Verification items for the finished model (mm, model axes). A direction names the side the tool comes from. Round coordinates to 2 decimals unless told otherwise and drop trailing zeros. Write each loop counter-clockwise with the first axis right and the second up, starting at its lowest first coordinate (ties: lowest second). Pieces come first, ordered by that corner, then holes. Notation, with made-up numbers: M 26,55 L 42,55 A21 cw 42,84 Z; hole C 24.5,-32 d8. An arc over 180 degrees is marked long. Write each question's results on one line, items separated by ' | '.
from build123d import *

# Parameters (mm, degrees)
PAD_DEPTH       = 250
POCKET_DEPTH    = 2
POCKET001_DEPTH = 3


with BuildPart() as part:
    # Sketch → Pad (new body)
    with BuildSketch(Plane.XZ):
        Polygon((0, 0), (-15, 0), (-15, 1.5), (-14, 1.5), (-14, 5.5), (-17.5, 6.5), (-17.5, 7.5), (-12.5, 7.5), (-12.5, 1.5), (0, 1.5), (12.5, 1.5), (12.5, 7.5), (17.5, 7.5), (17.51485, 6.5), (14, 5.5), (14, 1.5), (15, 1.5), (15, 0), align=None)
    extrude(amount=PAD_DEPTH)

    # Sketch001 (on Face10 of Pad) → Pocket (cut)
    with BuildSketch(Plane(origin=(0, 0, 1.5), x_dir=(-1, 0, 0), z_dir=(0, 0, 1))):
        with BuildLine():
            ThreePointArc((2.5, 2.5), (0, 5), (-2.5, 2.5))
            Line((-2.5, 2.5), (-2.5, -2.5))
            ThreePointArc((-2.5, -2.5), (0, -5), (2.5, -2.5))
            Line((2.5, 2.5), (2.5, -2.5))
        make_face()
        with BuildLine():
            ThreePointArc((2.5, 15), (0, 17.5), (-2.5, 15))
            Line((-2.5, 15), (-2.5, 10))
            ThreePointArc((-2.5, 10), (0, 7.5), (2.5, 10))
            Line((2.5, 15), (2.5, 10))
        make_face()
        with BuildLine():
            ThreePointArc((2.5, 27.5), (0, 30), (-2.5, 27.5))
            Line((-2.5, 27.5), (-2.5, 22.5))
            ThreePointArc((-2.5, 22.5), (0, 20), (2.5, 22.5))
            Line((2.5, 27.5), (2.5, 22.5))
        make_face()
        with BuildLine():
            ThreePointArc((2.5, 40), (0, 42.5), (-2.5, 40))
            Line((-2.5, 40), (-2.5, 35))
            ThreePointArc((-2.5, 35), (0, 32.5), (2.5, 35))
            Line((2.5, 40), (2.5, 35))
        make_face()
        with BuildLine():
            ThreePointArc((2.5, 52.5), (0, 55), (-2.5, 52.5))
            Line((-2.5, 52.5), (-2.5, 47.5))
            ThreePointArc((-2.5, 47.5), (0, 45), (2.5, 47.5))
            Line((2.5, 52.5), (2.5, 47.5))
        make_face()
        with BuildLine():
            ThreePointArc((2.5, 65), (0, 67.5), (-2.5, 65))
            Line((-2.5, 65), (-2.5, 60))
            ThreePointArc((-2.5, 60), (0, 57.5), (2.5, 60))
            Line((2.5, 65), (2.5, 60))
        make_face()
        with BuildLine():
            ThreePointArc((2.5, 77.5), (0, 80), (-2.5, 77.5))
            Line((-2.5, 77.5), (-2.5, 72.5))
            ThreePointArc((-2.5, 72.5), (0, 70), (2.5, 72.5))
            Line((2.5, 77.5), (2.5, 72.5))
        make_face()
        with BuildLine():
            ThreePointArc((2.5, 90), (0, 92.5), (-2.5, 90))
            Line((-2.5, 90), (-2.5, 85))
            ThreePointArc((-2.5, 85), (0, 82.5), (2.5, 85))
            Line((2.5, 90), (2.5, 85))
        make_face()
        with BuildLine():
            ThreePointArc((2.5, 102.5), (0, 105), (-2.5, 102.5))
            Line((-2.5, 102.5), (-2.5, 97.5))
            ThreePointArc((-2.5, 97.5), (0, 95), (2.5, 97.5))
            Line((2.5, 102.5), (2.5, 97.5))
        make_face()
        with BuildLine():
            ThreePointArc((2.5, 115), (0, 117.5), (-2.5, 115))
            Line((-2.5, 115), (-2.5, 110))
            ThreePointArc((-2.5, 110), (0, 107.5), (2.5, 110))
            Line((2.5, 115), (2.5, 110))
        make_face()
        with BuildLine():
            ThreePointArc((2.5, 127.5), (0, 130), (-2.5, 127.5))
            Line((-2.5, 127.5), (-2.5, 122.5))
            ThreePointArc((-2.5, 122.5), (0, 120), (2.5, 122.5))
            Line((2.5, 127.5), (2.5, 122.5))
        make_face()
        with BuildLine():
            ThreePointArc((2.5, 140), (0, 142.5), (-2.5, 140))
            Line((-2.5, 140), (-2.5, 135))
            ThreePointArc((-2.5, 135), (0, 132.5), (2.5, 135))
            Line((2.5, 140), (2.5, 135))
        make_face()
        with BuildLine():
            ThreePointArc((2.5, 152.5), (0, 155), (-2.5, 152.5))
            Line((-2.5, 152.5), (-2.5, 147.5))
            ThreePointArc((-2.5, 147.5), (0, 145), (2.5, 147.5))
            Line((2.5, 152.5), (2.5, 147.5))
        make_face()
        with BuildLine():
            ThreePointArc((2.5, 165), (0, 167.5), (-2.5, 165))
            Line((-2.5, 165), (-2.5, 160))
            ThreePointArc((-2.5, 160), (0, 157.5), (2.5, 160))
            Line((2.5, 165), (2.5, 160))
        make_face()
        with BuildLine():
            ThreePointArc((2.5, 177.5), (0, 180), (-2.5, 177.5))
            Line((-2.5, 177.5), (-2.5, 172.5))
            ThreePointArc((-2.5, 172.5), (0, 170), (2.5, 172.5))
            Line((2.5, 177.5), (2.5, 172.5))
        make_face()
        with BuildLine():
            ThreePointArc((2.5, 190), (0, 192.5), (-2.5, 190))
            Line((-2.5, 190), (-2.5, 185))
            ThreePointArc((-2.5, 185), (0, 182.5), (2.5, 185))
            Line((2.5, 190), (2.5, 185))
        make_face()
        with BuildLine():
            ThreePointArc((2.5, 202.5), (0, 205), (-2.5, 202.5))
            Line((-2.5, 202.5), (-2.5, 197.5))
            ThreePointArc((-2.5, 197.5), (0, 195), (2.5, 197.5))
            Line((2.5, 202.5), (2.5, 197.5))
        make_face()
        with BuildLine():
            ThreePointArc((2.5, 215), (0, 217.5), (-2.5, 215))
            Line((-2.5, 215), (-2.5, 210))
            ThreePointArc((-2.5, 210), (0, 207.5), (2.5, 210))
            Line((2.5, 215), (2.5, 210))
        make_face()
        with BuildLine():
            ThreePointArc((2.5, 227.5), (0, 230), (-2.5, 227.5))
            Line((-2.5, 227.5), (-2.5, 222.5))
            ThreePointArc((-2.5, 222.5), (0, 220), (2.5, 222.5))
            Line((2.5, 227.5), (2.5, 222.5))
        make_face()
        with BuildLine():
            ThreePointArc((2.5, 240), (0, 242.5), (-2.5, 240))
            Line((-2.5, 240), (-2.5, 235))
            ThreePointArc((-2.5, 235), (0, 232.5), (2.5, 235))
            Line((2.5, 240), (2.5, 235))
        make_face()
        with BuildLine():
            ThreePointArc((2.5, 252.5), (0, 255), (-2.5, 252.5))
            Line((-2.5, 252.5), (-2.5, 247.5))
            ThreePointArc((-2.5, 247.5), (0, 245), (2.5, 247.5))
            Line((2.5, 252.5), (2.5, 247.5))
        make_face()
        with BuildLine():
            ThreePointArc((2.5, 265), (0, 267.5), (-2.5, 265))
            Line((-2.5, 265), (-2.5, 260))
            ThreePointArc((-2.5, 260), (0, 257.5), (2.5, 260))
            Line((2.5, 265), (2.5, 260))
        make_face()
        with BuildLine():
            ThreePointArc((2.5, 277.5), (0, 280), (-2.5, 277.5))
            Line((-2.5, 277.5), (-2.5, 272.5))
            ThreePointArc((-2.5, 272.5), (0, 270), (2.5, 272.5))
            Line((2.5, 277.5), (2.5, 272.5))
        make_face()
        with BuildLine():
            ThreePointArc((-2.5, 285), (0, 282.5), (2.5, 285))
            Line((2.5, 285), (2.5, 290))
            ThreePointArc((2.5, 290), (0, 292.5), (-2.5, 290))
            Line((-2.5, 285), (-2.5, 290))
        make_face()
    extrude(amount=-POCKET_DEPTH, mode=Mode.SUBTRACT)

    # Sketch001 (on Face10 of Pad) → Pocket001 (cut)
    with BuildSketch(Plane(origin=(0, 0, 1.5), x_dir=(-1, 0, 0), z_dir=(0, 0, 1))):
        with BuildLine():
            ThreePointArc((2.5, 2.5), (0, 5), (-2.5, 2.5))
            Line((-2.5, 2.5), (-2.5, -2.5))
            ThreePointArc((-2.5, -2.5), (0, -5), (2.5, -2.5))
            Line((2.5, 2.5), (2.5, -2.5))
        make_face()
        with BuildLine():
            ThreePointArc((2.5, 15), (0, 17.5), (-2.5, 15))
            Line((-2.5, 15), (-2.5, 10))
            ThreePointArc((-2.5, 10), (0, 7.5), (2.5, 10))
            Line((2.5, 15), (2.5, 10))
        make_face()
        with BuildLine():
            ThreePointArc((2.5, 27.5), (0, 30), (-2.5, 27.5))
            Line((-2.5, 27.5), (-2.5, 22.5))
            ThreePointArc((-2.5, 22.5), (0, 20), (2.5, 22.5))
            Line((2.5, 27.5), (2.5, 22.5))
        make_face()
        with BuildLine():
            ThreePointArc((2.5, 40), (0, 42.5), (-2.5, 40))
            Line((-2.5, 40), (-2.5, 35))
            ThreePointArc((-2.5, 35), (0, 32.5), (2.5, 35))
            Line((2.5, 40), (2.5, 35))
        make_face()
        with BuildLine():
            ThreePointArc((2.5, 52.5), (0, 55), (-2.5, 52.5))
            Line((-2.5, 52.5), (-2.5, 47.5))
            ThreePointArc((-2.5, 47.5), (0, 45), (2.5, 47.5))
            Line((2.5, 52.5), (2.5, 47.5))
        make_face()
        with BuildLine():
            ThreePointArc((2.5, 65), (0, 67.5), (-2.5, 65))
            Line((-2.5, 65), (-2.5, 60))
            ThreePointArc((-2.5, 60), (0, 57.5), (2.5, 60))
            Line((2.5, 65), (2.5, 60))
        make_face()
        with BuildLine():
            ThreePointArc((2.5, 77.5), (0, 80), (-2.5, 77.5))
            Line((-2.5, 77.5), (-2.5, 72.5))
            ThreePointArc((-2.5, 72.5), (0, 70), (2.5, 72.5))
            Line((2.5, 77.5), (2.5, 72.5))
        make_face()
        with BuildLine():
            ThreePointArc((2.5, 90), (0, 92.5), (-2.5, 90))
            Line((-2.5, 90), (-2.5, 85))
            ThreePointArc((-2.5, 85), (0, 82.5), (2.5, 85))
            Line((2.5, 90), (2.5, 85))
        make_face()
        with BuildLine():
            ThreePointArc((2.5, 102.5), (0, 105), (-2.5, 102.5))
            Line((-2.5, 102.5), (-2.5, 97.5))
            ThreePointArc((-2.5, 97.5), (0, 95), (2.5, 97.5))
            Line((2.5, 102.5), (2.5, 97.5))
        make_face()
        with BuildLine():
            ThreePointArc((2.5, 115), (0, 117.5), (-2.5, 115))
            Line((-2.5, 115), (-2.5, 110))
            ThreePointArc((-2.5, 110), (0, 107.5), (2.5, 110))
            Line((2.5, 115), (2.5, 110))
        make_face()
        with BuildLine():
            ThreePointArc((2.5, 127.5), (0, 130), (-2.5, 127.5))
            Line((-2.5, 127.5), (-2.5, 122.5))
            ThreePointArc((-2.5, 122.5), (0, 120), (2.5, 122.5))
            Line((2.5, 127.5), (2.5, 122.5))
        make_face()
        with BuildLine():
            ThreePointArc((2.5, 140), (0, 142.5), (-2.5, 140))
            Line((-2.5, 140), (-2.5, 135))
            ThreePointArc((-2.5, 135), (0, 132.5), (2.5, 135))
            Line((2.5, 140), (2.5, 135))
        make_face()
        with BuildLine():
            ThreePointArc((2.5, 152.5), (0, 155), (-2.5, 152.5))
            Line((-2.5, 152.5), (-2.5, 147.5))
            ThreePointArc((-2.5, 147.5), (0, 145), (2.5, 147.5))
            Line((2.5, 152.5), (2.5, 147.5))
        make_face()
        with BuildLine():
            ThreePointArc((2.5, 165), (0, 167.5), (-2.5, 165))
            Line((-2.5, 165), (-2.5, 160))
            ThreePointArc((-2.5, 160), (0, 157.5), (2.5, 160))
            Line((2.5, 165), (2.5, 160))
        make_face()
        with BuildLine():
            ThreePointArc((2.5, 177.5), (0, 180), (-2.5, 177.5))
            Line((-2.5, 177.5), (-2.5, 172.5))
            ThreePointArc((-2.5, 172.5), (0, 170), (2.5, 172.5))
            Line((2.5, 177.5), (2.5, 172.5))
        make_face()
        with BuildLine():
            ThreePointArc((2.5, 190), (0, 192.5), (-2.5, 190))
            Line((-2.5, 190), (-2.5, 185))
            ThreePointArc((-2.5, 185), (0, 182.5), (2.5, 185))
            Line((2.5, 190), (2.5, 185))
        make_face()
        with BuildLine():
            ThreePointArc((2.5, 202.5), (0, 205), (-2.5, 202.5))
            Line((-2.5, 202.5), (-2.5, 197.5))
            ThreePointArc((-2.5, 197.5), (0, 195), (2.5, 197.5))
            Line((2.5, 202.5), (2.5, 197.5))
        make_face()
        with BuildLine():
            ThreePointArc((2.5, 215), (0, 217.5), (-2.5, 215))
            Line((-2.5, 215), (-2.5, 210))
            ThreePointArc((-2.5, 210), (0, 207.5), (2.5, 210))
            Line((2.5, 215), (2.5, 210))
        make_face()
        with BuildLine():
            ThreePointArc((2.5, 227.5), (0, 230), (-2.5, 227.5))
            Line((-2.5, 227.5), (-2.5, 222.5))
            ThreePointArc((-2.5, 222.5), (0, 220), (2.5, 222.5))
            Line((2.5, 227.5), (2.5, 222.5))
        make_face()
        with BuildLine():
            ThreePointArc((2.5, 240), (0, 242.5), (-2.5, 240))
            Line((-2.5, 240), (-2.5, 235))
            ThreePointArc((-2.5, 235), (0, 232.5), (2.5, 235))
            Line((2.5, 240), (2.5, 235))
        make_face()
        with BuildLine():
            ThreePointArc((2.5, 252.5), (0, 255), (-2.5, 252.5))
            Line((-2.5, 252.5), (-2.5, 247.5))
            ThreePointArc((-2.5, 247.5), (0, 245), (2.5, 247.5))
            Line((2.5, 252.5), (2.5, 247.5))
        make_face()
        with BuildLine():
            ThreePointArc((2.5, 265), (0, 267.5), (-2.5, 265))
            Line((-2.5, 265), (-2.5, 260))
            ThreePointArc((-2.5, 260), (0, 257.5), (2.5, 260))
            Line((2.5, 265), (2.5, 260))
        make_face()
        with BuildLine():
            ThreePointArc((2.5, 277.5), (0, 280), (-2.5, 277.5))
            Line((-2.5, 277.5), (-2.5, 272.5))
            ThreePointArc((-2.5, 272.5), (0, 270), (2.5, 272.5))
            Line((2.5, 277.5), (2.5, 272.5))
        make_face()
        with BuildLine():
            ThreePointArc((-2.5, 285), (0, 282.5), (2.5, 285))
            Line((2.5, 285), (2.5, 290))
            ThreePointArc((2.5, 290), (0, 292.5), (-2.5, 290))
            Line((-2.5, 285), (-2.5, 290))
        make_face()
    extrude(amount=-POCKET001_DEPTH, mode=Mode.SUBTRACT)


solid = part.part
1) Access from +Z, -Z, +X, -X, +Y, -Y to the whole of each face (thin tool, end or side, straight path). Record for faces 4 (the flat face through (-3, -123, 1.5)), 5 (the flat face through (14, -123, 4)), 6 (the flat face through (15, -123, 7.5)).
Calculated:
face 4: +Z, +Y, -Y | face 5: +X, +Y, -Y | face 6: +Z, +X, -X, +Y, -Y
2) Sectioned sample at D-D, the plane x = 9. Record the cut outline in (y, z).
Calculated:
outline: M -250,0 L 0,0 L 0,1.5 L -250,1.5 Z
3) Material ranges on line 1 (X direction, y = -180, z = 7.25); line 2 (X direction, y = -69.5, z = 1.75); line 3 (Z direction, x = -8, y = -26.5), recorded low to high. Write a range as [from, to].
Calculated:
line 1: x = [-17.5, -12.5], [12.5, 17.5] | line 2: x = [-14, -12.5], [12.5, 14] | line 3: z = [0, 1.5]
4) Sectioned sample at A-A, the plane y = -75. Record the cut outline in (x, z).
Calculated:
outline: M -17.5,6.5 L -14,5.5 L -14,1.5 L -15,1.5 L -15,0 L -2.5,0 L -2.5,1.5 L -12.5,1.5 L -12.5,7.5 L -17.5,7.5 Z; M 2.5,0 L 15,0 L 15,1.5 L 14,1.5 L 14,5.5 L 17.51,6.5 L 17.5,7.5 L 12.5,7.5 L 12.5,1.5 L 2.5,1.5 Z
5) Sectioned sample at B-B, the plane z = 4. Record the cut outline in (x, y).
Calculated:
outline: M -14,-250 L -12.5,-250 L -12.5,0 L -14,0 Z; M 12.5,-250 L 14,-250 L 14,0 L 12.5,0 Z
6) Sectioned sample at C-C, the plane x = 0. Count the separate pieces of the cut face and the enclosed holes in it, and give its area (3 significant figures).
Calculated:
separate pieces: 20 | enclosed holes: 0 | area: 75.0 mm²
7) Depth check by flat-ended pin: P1, Ø1.6, axis at y = -75.5, z = 1, coming from the -X side; P2, Ø5, axis at x = 9.5, y = -95, coming from the +Z side; P3, Ø1.6, axis at y = -176, z = 1, coming from the +X side. Enter the tip coordinate at first touch or a pass-through.
Calculated:
P1: stops at x = -15 | P2: stops at z = 1.5 | P3: stops at x = 15
8) Draft check along Z on faces 1 (the flat face through (-14, -123, 3)), 2 (the flat face through (12.5, -123, 4)), 3 (the flat face through (-15, -123, 7.5)). Enter one of: pulls with the +Z half, pulls with the -Z half, needs draft (parallel to the pull), parting line crosses it, or undercut.
Calculated:
face 1: undercut | face 2: needs draft | face 3: pulls with the +Z half
